The model under review builds one solid part; all positions refer to its coordinate system, in mm. A direction names the side the tool comes from. Coordinates: 2 decimals unless noted, no trailing zeros. Write each loop counter-clockwise with the first axis right and the second up, starting at its lowest first coordinate (ties: lowest second). Pieces come first, ordered by that corner, then holes.
Autodesk Inventor part; units mm, degrees
ref_plane "YZ Plane" through (0, 0, 0) normal (1, 0, 0) x (0, 1, 0)
ref_plane "XZ Plane" through (0, 0, 0) normal (0, 1, 0) x (-1, 0, 0)
ref_plane "XY Plane" through (0, 0, 0) normal (0, 0, 1) x (1, 0, 0)
sketch "Sketch1" plane through (0, 0, 0) normal (0, 0, 1) x (1, 0, 0)
  circle A0 centre (0, 0) radius 10
  circle A1 centre (0, 0) radius 11
  circle A2 centre (0, 0) radius 15
  dimension "d0" = 20
  dimension "d1" = 22
  dimension "d2" = 30
extrude "Extrusion1" add sketch "Sketch1" along normal blind 28 contours A0 | A1 | A2
extrude "Extrusion2" cut sketch "Sketch1" along normal blind 12 contours A1
extrude "Extrusion3" cut sketch "Sketch1" along normal blind 27 contours A0
sketch "Sketch2" plane through (0, 0, 0) normal (1, 0, 0) x (0, 1, 0)
  line L0 (15, 28) -> (-15, 28)
  line L1 (15, 0) -> (-15, 0)
  circle A0 centre (0, 16) radius 2.5
  point P0 (0, 0)
  point P1 (0, 0)
  dimension "d9" = 5
  dimension "d10" = 16
extrude "Extrusion4" cut sketch "Sketch2" along normal through all both and the other way through all
chamfer "Chamfer1" distance 0.5 angle 45 2 edges at (-11, 0, 0) (-15, 0, 0)
chamfer "Chamfer2" distance 0.1 angle 45 4 edges at (14.7902, -2.5, 16.0004) (14.8791, 1.901, 14.3764) (14.8788, 1.9027, 17.6217) (-14.7902, -2.4999, 15.9815)
properties part number "Piston"
Item 1: Machinability: for faces 1 (the face through (0, 0, 28)), 2 (the face through (9.54, -3, 19.4)), which of the approach directions +Z, -Z, +X, -X, +Y, -Y give a long, thin tool a straight path to every point of the face, cutting with its end or side? Answer none if there is none.
Solved:
face 1: +Z, +X, -X, +Y, -Y
face 2: -Z
Item 2: Take a section at B-B, the plane x = 0. Write out the cut boundary in (y, z), plus the area to 4 significant figures.
Solved:
outline: (-15, 0.5) - (-14.5, 0) - (-11.5, 0) - (-11, 0.5) - (-11, 12) - (-10, 12) - (-10, 27) - (10, 27) - (10, 12) - (11, 12) - (11, 0.5) - (11.5, 0) - (14.5, 0) - (15, 0.5) - (15, 28) - (-15, 28) - close
area: 275.5 mm2
Item 3: Mouldability with a two-part tool opening along Y and no side actions: class faces 3 (the face through (-2.38, 10.74, 6.17)), 4 (the face through (-9, 8, 0)), 5 (the face through (-12.25, 2.31, 15.04)), 6 (the face through (13.856, 5.745, 14.058)) as pulls with the +Y half, pulls with the -Y half, needs draft (parallel to the pull), parting line crosses it, or undercut.
Solved:
face 3: undercut
face 4: needs draft
face 5: undercut
face 6: parting line crosses it
Item 4: Take a section at A-A, the plane z = 26. Write out the cut boundary in (x, y).
Solved:
outline: circle Ø30 at (0, 0); hole circle Ø20 at (0, 0)
Item 5: Take a section at C-C, the plane z = 7.25. Write out the cut boundary in (x, y).
Solved:
outline: circle Ø30 at (0, 0); hole circle Ø22 at (0, 0)
Item 6: To check wall thickness, follow line 1 along Y through (x, z) = (0, 16.25); line 2 along Y through (x, z) = (0, 4); line 3 along Z through (x, y) = (12, 0). State the ranges of each line that lie inside material, in increasing order.
Solved:
line 1: y = -15 to -10, 10 to 15
line 2: y = -15 to -11, 11 to 15
line 3: z = 0 to 13.5, 18.5 to 28
Item 7: For pin 1 (1.5 mm diameter, centred on y = 1.5, z = 11, fed in from +X); pin 2 (10 mm diameter, centred on x = 9.5, z = 21, fed in from +Y); pin 3 (10 mm diameter, centred on y = -8.5, z = 14.5, fed in from +X), all flat-tipped, find the tip position at first contact; note any pin that passes through.
Solved:
pin 1: stops at x = 14.98
pin 2: stops at y = 14.31
pin 3: stops at x = 14.59
